from build123d import *

# Parameters (mm, degrees)
F1_R     = 38.1
F2_DEPTH = 15.2828320861
F3_R     = 23.1262571724
F4_DEPTH = 25.4
F5_R     = 38.1
F5_R_2   = 31.75
F6_DEPTH = 25.4


# Not quite as in the source:
# - a feature names something its author has since deleted; it is built from what else it names


with BuildPart() as f2:
    # F1 (on offset) → F2 (new body)
    with BuildSketch(Plane.XY.offset(-83.2833182067)):
        Circle(F1_R)
    extrude(amount=-F2_DEPTH)

    # F3 (on face) → F4 (cut)
    with BuildSketch(Plane.XY.offset(-83.2833182067)):
        Circle(F3_R)
    extrude(amount=-F4_DEPTH, mode=Mode.SUBTRACT)

    # F5 (on face) → F6 (join)
    with BuildSketch(Plane(origin=(0, 0, -98.5661502928), x_dir=(1, 0, 0), z_dir=(0, 0, -1))):
        Circle(F5_R)
        Circle(F5_R_2, mode=Mode.SUBTRACT)
    extrude(amount=F6_DEPTH)


solid = f2.part
For this review, take the finished solid that the model builds, in its own axes (mm). A direction names the side the tool comes from. Give positions to 0.01 mm unless a question says otherwise; leave off trailing zeros. Loops run counter-clockwise (first coordinate to the right, second up) from the corner with the lowest first, then second, coordinate; pieces in that order, holes last. Notation, with made-up numbers: M 28,52 L 49,52 A15 ccw 49,69 Z; hole C 23.25,46 d7. An arc over 180 degrees is marked long. Put each result on its own line as item: value. Start each with the question number.
(1) The part is to be moulded in two halves that separate along X. For faces 1 (the cylindrical face through (-30.235, 23.183, -103.34)), 2 (the flat face through (2.2, -23.4, -98.566)), 3 (the flat face through (-1, -25, -83.283)), say which applies: +X half, -X half, draft (parallel to the pull), parting line (faces both ways), or undercut.
(2) Add section C-C, the plane z = -119.5. Write out the cut boundary in (x, y), then the cut area to 3 significant figures.
(3) For pin 1 (6 mm diameter, centred on x = -2, y = -24.5, fed in from -Z); pin 2 (3 mm diameter, centred on y = 21, z = -105, fed in from +X); pin 3 (1.5 mm diameter, centred on y = -27.5, z = -108.5, fed in from +X), all flat-tipped, find the tip position at first contact; note any pin that passes through.
(4) Add section D-D, the plane x = 27.5. Write out the cut boundary in (y, z), then the cut area to 3 significant figures.
(5) Wall thickness on L1, parallel to Y at x = 0, z = -112; L2, parallel to Y at x = 0, z = -90.25; L3, parallel to X at y = 27, z = -105: over which ranges is each line inside the solid? List them lowest first.
(6) Add section A-A, the plane x = 0. Write out the cut boundary in (y, z).
(7) Machinability: for faces 4 (the cylindrical face through (10.7, -20.5, -90.8)), 5 (the cylindrical face through (-6.883, 30.995, -111.088)), which of the approach directions +Z, -Z, +X, -X, +Y, -Y give a long, thin tool a straight path to every point of the face, cutting with its end or side? Answer none if there is none.
Result:
1. face 1: parting line
1. face 2: undercut
1. face 3: draft
2. outline: C 0,0 d76.2; hole C 0,0 d63.5
2. area: 1,390 mm^2
3. pin 1: stops at z = -98.57
3. pin 2: stops at x = 32.73
3. pin 3: stops at x = 27.13
4. outline: M -26.37,-123.97 L -15.87,-123.97 L -15.87,-98.57 L 15.87,-98.57 L 15.87,-123.97 L 26.37,-123.97 L 26.37,-83.28 L -26.37,-83.28 Z
4. area: 1,340 mm^2
5. L1: y = -38.1 to -31.75, 31.75 to 38.1
5. L2: y = -38.1 to -23.13, 23.13 to 38.1
5. L3: x = -26.88 to -16.71, 16.71 to 26.88
6. outline: M -38.1,-123.97 L -31.75,-123.97 L -31.75,-98.57 L -23.13,-98.57 L -23.13,-83.28 L -38.1,-83.28 Z; M 23.13,-98.57 L 31.75,-98.57 L 31.75,-123.97 L 38.1,-123.97 L 38.1,-83.28 L 23.13,-83.28 Z
7. face 4: +Z, -Z
7. face 5: -Z
